from build123d import *

# Parameters (mm, degrees)
F0_R     = 7.943812
F1_DEPTH = 20.066
F2_DEPTH = 46.736


with BuildPart() as f1:
    # F0 (on Front) → F1 (new body)
    with BuildSketch(Plane.XZ):
        with BuildLine():
            Line((17.78, -34.318883), (17.78, 34.318883))
            ThreePointArc((17.78, 34.318883), (0, 52.098883), (-17.78, 34.318883))
            Line((-17.78, 34.318883), (-17.78, -34.318883))
            ThreePointArc((-17.78, -34.318883), (0, -16.538883), (17.78, -34.318883))
        make_face()
        with Locations((0, 34.318883)):
            Circle(F0_R, mode=Mode.SUBTRACT)
        with BuildLine():
            ThreePointArc((-17.78, -34.318883), (0, -52.098883), (17.78, -34.318883))
            ThreePointArc((17.78, -34.318883), (0, -16.538883), (-17.78, -34.318883))
        make_face()
        with Locations((0, -34.318883)):
            Circle(F0_R, mode=Mode.SUBTRACT)
    extrude(amount=F1_DEPTH)

    # F0 (on Front) → F2 (join)
    with BuildSketch(Plane.XZ):
        with BuildLine():
            ThreePointArc((-17.78, -34.318883), (0, -52.098883), (17.78, -34.318883))
            ThreePointArc((17.78, -34.318883), (0, -16.538883), (-17.78, -34.318883))
        make_face()
        with Locations((0, -34.318883)):
            Circle(F0_R, mode=Mode.SUBTRACT)
    extrude(amount=F2_DEPTH)

    # F4: F1 across plane


with BuildPart() as f1_1:
    add(f1.part)
    add(f1.part.mirror(Plane(origin=(0, -46.736, -34.318883), x_dir=(1, 0, 0), z_dir=(0, -1, 0))))


solid = f1_1.part
Design review of the part built by this model. Coordinates are the model's own, in mm. A direction names the side the tool comes from. Give positions to 0.01 mm unless a question says otherwise; leave off trailing zeros. Loops run counter-clockwise (first coordinate to the right, second up) from the corner with the lowest first, then second, coordinate; pieces in that order, holes last. Notation, with made-up numbers: (-24, 70.25) - (8, 70.25) arc R30 ccw to (8, 108.25) - close; hole circle Ø4 at (53.5, 26.25). An arc over 180 degrees is marked (long way). Use CSV: the item, a comma, the result in double quotes. Start each with the question number.
1. Add section D-D (x = -11). State the section outline as (y, z) points, plus the area to 3 significant figures.
2. Insertion check: P1, Ø5, axis at x = -3.5, y = -67.5, coming from the +Z side; P2, Ø1.5, axis at y = -56.5, z = -40, coming from the -X side; P3, Ø8, axis at x = -9.5, y = -68.5, coming from the +Z side. Each pin has a flat end and moves straight along its axis. Give the tip position at first contact, or say it passes through.
3. Add section A-A (x = 0). State the section outline as (y, z) points.
4. Add section C-C (z = -14.5). State the section outline as (x, y) points, plus the area to 3 significant figures.
5. Add section B-B (y = -79). State the section outline as (x, z) points, plus the area to 3 significant figures.
6. Wall thickness on L1, parallel to Z at x = 0, y = -6; L2, parallel to Y at x = 16.5, z = 0; L3, parallel to Z at x = 5.5, y = -40: over which ranges is each line inside the solid? List them lowest first.
7. Draft analysis for pull direction X (two halves, no side actions). For faces 3 (the flat face through (0, -93.472, 1)), 4 (the cylindrical face through (-1.722, -9.893, 26.564)), 5 (the flat face through (17.78, -10, 0)), state which applies: released by +X, released by -X, zero draft, split by the parting line, or undercut.
8. Machinability: for faces 1 (the cylindrical face through (8.204, -47.39, -50.093)), 2 (the flat face through (-17.78, -10, 0)), which of the approach directions +Z, -Z, +X, -X, +Y, -Y give a long, thin tool a straight path to every point of the face, cutting with its end or side? Answer none if there is none.
Results found:
1,outline,"(-93.47, -48.29) - (0, -48.29) - (0, 48.29) - (-20.07, 48.29) - (-20.07, -20.35) - (-73.41, -20.35) - (-73.41, 48.29) - (-93.47, 48.29) - close"
1,area,"5,370 mm²"
2,P1,"stops at z = -16.57"
2,P2,"stops at x = -17.08"
2,P3,"stops at z = -17.41"
3,outline,"(-93.47, -52.1) - (0, -52.1) - (0, -42.26) - (-93.47, -42.26) - close; (-93.47, -26.38) - (0, -26.38) - (0, 26.38) - (-20.07, 26.38) - (-20.07, -16.54) - (-73.41, -16.54) - (-73.41, 26.38) - (-93.47, 26.38) - close; (-93.47, 42.26) - (-73.41, 42.26) - (-73.41, 52.1) - (-93.47, 52.1) - close; (-20.07, 42.26) - (0, 42.26) - (0, 52.1) - (-20.07, 52.1) - close"
4,outline,"(-17.78, -93.47) - (17.78, -93.47) - (17.78, -73.41) - (-17.78, -73.41) - close; (-17.78, -20.07) - (17.78, -20.07) - (17.78, 0) - (-17.78, 0) - close"
4,area,"1,430 mm²"
5,outline,"(-17.78, -34.32) arc R17.78 ccw to (17.78, -34.32) - (17.78, 34.32) arc R17.78 ccw to (-17.78, 34.32) - close; hole circle Ø15.89 at (0, -34.32); hole circle Ø15.89 at (0, 34.32)"
5,area,"3,040 mm²"
6,L1,"z = -52.1 to -42.26, -26.38 to 26.38, 42.26 to 52.1"
6,L2,"y = -93.47 to -73.41, -20.07 to 0"
6,L3,"z = -51.23 to -40.05, -28.59 to -17.41"
7,face 3,"zero draft"
7,face 4,"undercut"
7,face 5,"released by +X"
8,face 1,"none"
8,face 2,"+Z, -Z, -X, +Y, -Y"
